Check sheet for the modelled part. Datum: model origin and axes. Units: mm. A direction names the side the tool comes from. Round coordinates to 2 decimals unless told otherwise and drop trailing zeros. Write each loop counter-clockwise with the first axis right and the second up, starting at its lowest first coordinate (ties: lowest second). Pieces come first, ordered by that corner, then holes. Notation, with made-up numbers: M 19.25,-16 L 57.25,-16 A26 cw 57.25,16 Z; hole C 36.5,69.5 d8. An arc over 180 degrees is marked long. One line per item, written item: value.
from build123d import *

# Parameters (mm, degrees)
SKETCH1_W           = 140
SKETCH1_H           = 140
BOSS_EXTRUDE1_DEPTH = 3
SKETCH2_W           = 39.5
SKETCH2_H           = 3
SKETCH2_W_2         = 29
CUT_EXTRUDE2_DEPTH  = 3
SKETCH4_W           = 3
SKETCH4_H           = 16
CUT_EXTRUDE3_DEPTH  = 3


with BuildPart() as part:
    # Sketch1 → Boss-Extrude1 (new body)
    with BuildSketch(Plane(origin=(0, 0, 0), x_dir=(1, 0, 0), z_dir=(0, 1, 0))):
        Rectangle(SKETCH1_W, SKETCH1_H)
    extrude(amount=BOSS_EXTRUDE1_DEPTH)

    # Sketch2 → Cut-Extrude2 (cut)
    with BuildSketch(Plane(origin=(0, 3, 0), x_dir=(1, 0, 0), z_dir=(0, 1, 0))):
        with Locations((-50.25, 68.5)):
            Rectangle(SKETCH2_W, SKETCH2_H)
        with Locations((-50.25, -68.5)):
            Rectangle(SKETCH2_W, SKETCH2_H)
        with Locations((50.25, -68.5)):
            Rectangle(SKETCH2_W, SKETCH2_H)
        with Locations((50.25, 68.5)):
            Rectangle(SKETCH2_W, SKETCH2_H)
        with Locations((0, 68.5)):
            Rectangle(SKETCH2_W_2, SKETCH2_H)
        with Locations((0, -68.5)):
            Rectangle(SKETCH2_W_2, SKETCH2_H)
    extrude(amount=-CUT_EXTRUDE2_DEPTH, mode=Mode.SUBTRACT)

    # Sketch4 → Cut-Extrude3 (cut)
    with BuildSketch(Plane(origin=(0, 3, 0), x_dir=(1, 0, 0), z_dir=(0, 1, 0))):
        with Locations((-68.5, 22.5)):
            Rectangle(SKETCH4_W, SKETCH4_H)
        with Locations((-68.5, -22.5)):
            Rectangle(SKETCH4_W, SKETCH4_H)
        with Locations((68.5, 22.5)):
            Rectangle(SKETCH4_W, SKETCH4_H)
        with Locations((68.5, -22.5)):
            Rectangle(SKETCH4_W, SKETCH4_H)
    extrude(amount=-CUT_EXTRUDE3_DEPTH, mode=Mode.SUBTRACT)


solid = part.part
Q1. Sectioned sample at B-B on x = -52. Enter the section's corners in (y, z).
Completed:
outline: M 0,-67 L 3,-67 L 3,67 L 0,67 Z
Q2. Scan line: line 1 (X direction, y = 2.05, z = 26). Record every from-to range of solid material in increasing order. Write a range as [from, to].
Completed:
line 1: [-67, 67]
Q3. Sectioned sample at A-A on z = 25. Enter the section's corners in (x, y), and give its area (3 significant figures).
Completed:
outline: M -67,0 L 67,0 L 67,3 L -67,3 Z
area: 402 mm^2
Q4. Access from +Z, -Z, +X, -X, +Y, -Y to the whole of each face (thin tool, end or side, straight path). Record for faces 4 (the flat face through (-30.5, 2, 69)), 5 (the flat face through (-51, 2, -67)), 6 (the flat face through (-67, 2, 23)), 7 (the flat face through (68, 2, -30.5)).
Completed:
face 4: +Z, -X, +Y, -Y
face 5: -Z, -X, +Y, -Y
face 6: -X, +Y, -Y
face 7: +X, +Y, -Y
Q5. Draft check along X on faces 1 (the flat face through (-69, 2, -14.5)), 2 (the flat face through (70, 1, 0)), 3 (the flat face through (14.5, 2, -68)). Enter one of: pulls with the +X half, pulls with the -X half, needs draft (parallel to the pull), parting line crosses it, or undercut.
Completed:
face 1: needs draft
face 2: pulls with the +X half
face 3: undercut
Q6. Depth check by flat-ended pin: P1, Ø1.5, axis at x = -68.5, y = 1, coming from the +Z side; P2, Ø1.5, axis at x = -68, y = 1.5, coming from the -Z side; P3, Ø0.9, axis at y = 1.5, z = -68, coming from the +X side. Enter the tip coordinate at first touch or a pass-through.
Completed:
P1: z = 67
P2: z = -67
P3: x = 30.5
